Source: CAD feature listing. Evaluate the final solid. Frame: model axes, mm. A direction names the side the tool comes from. Give positions to 0.01 mm unless a question says otherwise; leave off trailing zeros. Order: outer loops, then holes, each group sorted by start corner. A loop starts at its lowest first (then second) coordinate and runs counter-clockwise, first axis right, second up. Notation, with made-up numbers: (-6.5, 23) -> (44.5, 23) arc R23 cw to (44.5, 37) -> close; hole circle Ø10 at (13.25, 59.25). An arc over 180 degrees is marked (long way). Answer in a Markdown table with one row per item.
```python
from build123d import *

# Parameters (mm, degrees)
F1_DEPTH  = 64
F2_R      = 60
F3_DEPTH  = 28.5
F4_R      = 60
F4_R_2    = 57
F5_DEPTH  = 25.5
F7_DEPTH  = 6.25
F8_R      = 13.15
F9_DEPTH  = 64.001
F10_R     = 11
F11_DEPTH = 12
F12_R     = 13.15
F13_DEPTH = 25
F14_R     = 7
F15_DEPTH = 57.751


with BuildPart() as f1:
    # F0 (on Front) → F1 (new body)
    with BuildSketch(Plane.XZ):
        with BuildLine():
            ThreePointArc((-32.5, -28), (-25.1776695297, -45.6776695297), (-7.5, -53))
            Line((-7.5, -53), (7.5, -53))
            ThreePointArc((7.5, -53), (25.1776695297, -45.6776695297), (32.5, -28))
            Line((32.5, -28), (32.5, 28))
            ThreePointArc((32.5, 28), (25.1776695297, 45.6776695297), (7.5, 53))
            Line((7.5, 53), (-7.5, 53))
            ThreePointArc((-7.5, 53), (-25.1776695297, 45.6776695297), (-32.5, 28))
            Line((-32.5, 28), (-32.5, -28))
        make_face()
    extrude(amount=F1_DEPTH)

    # F2 (on face) → F3 (join)
    with BuildSketch(Plane.XZ.offset(64)):
        Circle(F2_R)
    extrude(amount=-F3_DEPTH)

    # F4 (on face) → F5 (cut)
    with BuildSketch(Plane.XZ.offset(64)):
        Circle(F4_R)
        Circle(F4_R_2, mode=Mode.SUBTRACT)
    extrude(amount=-F5_DEPTH, mode=Mode.SUBTRACT)

    # F6 (on face) → F7 (cut)
    with BuildSketch(Plane(origin=(0, 0, 0), x_dir=(-1, 0, 0), z_dir=(0, 1, 0))):
        with BuildLine():
            ThreePointArc((10.955166333, 46.2427935703), (16.0339049992, 39.9945133997), (17.85, 32.15))
            ThreePointArc((17.85, 32.15), (-7.8445133997, 16.1160950008), (-10.955166333, 46.2427935703))
            ThreePointArc((-10.955166333, 46.2427935703), (-10.6670838439, 46.4620865798), (-10.3746129282, 46.6754916127))
            add(Edge.make_bspline(
                [(-11.4193501695, 49.6480644458), (-9.7061666222, 49.8827470388), (-8.574372674, 48.2387921733), (-10.3746129282, 46.6754916127)],
                knots=[0, 0, 0, 0, 3.1442100344, 3.1442100344, 3.1442100344, 3.1442100344], degree=3))
            ThreePointArc((-11.4193501695, 49.6480644458), (-24.3852850691, 42.1027354841), (-29.5, 28))
            Line((-29.5, 28), (-29.5, -28))
            ThreePointArc((-29.5, -28), (-24.3852850691, -42.1027354841), (-11.4193501695, -49.6480644458))
            add(Edge.make_bspline(
                [(-11.4193501695, -49.6480644458), (-9.7061666222, -49.8827470388), (-8.574372674, -48.2387921733), (-10.3746129282, -46.6754916127)],
                knots=[0, 0, 0, 0, 3.1442100344, 3.1442100344, 3.1442100344, 3.1442100344], degree=3))
            ThreePointArc((-10.3746129282, -46.6754916127), (-10.6670838439, -46.4620865798), (-10.955166333, -46.2427935703))
            ThreePointArc((-10.955166333, -46.2427935703), (-7.8445133997, -16.1160950008), (17.85, -32.15))
            ThreePointArc((17.85, -32.15), (16.0339049992, -39.9945133997), (10.955166333, -46.2427935703))
            ThreePointArc((10.955166333, -46.2427935703), (10.6670838439, -46.4620865798), (10.3746129282, -46.6754916127))
            add(Edge.make_bspline(
                [(11.4193501695, -49.6480644458), (9.7061666222, -49.8827470388), (8.574372674, -48.2387921733), (10.3746129282, -46.6754916127)],
                knots=[0, 0, 0, 0, 3.1442100344, 3.1442100344, 3.1442100344, 3.1442100344], degree=3))
            ThreePointArc((11.4193501695, -49.6480644458), (24.3852850691, -42.1027354841), (29.5, -28))
            Line((29.5, -28), (29.5, 28))
            ThreePointArc((29.5, 28), (24.3852850691, 42.1027354841), (11.4193501695, 49.6480644458))
            add(Edge.make_bspline(
                [(11.4193501695, 49.6480644458), (9.7061666222, 49.8827470388), (8.574372674, 48.2387921733), (10.3746129282, 46.6754916127)],
                knots=[0, 0, 0, 0, 3.1442100344, 3.1442100344, 3.1442100344, 3.1442100344], degree=3))
            ThreePointArc((10.3746129282, 46.6754916127), (10.6670838439, 46.4620865798), (10.955166333, 46.2427935703))
        make_face()
    extrude(amount=-F7_DEPTH, mode=Mode.SUBTRACT)

    # F8 (on face) → F9 (cut, through all)
    with BuildSketch(Plane(origin=(0, 0, 0), x_dir=(-1, 0, 0), z_dir=(0, 1, 0))):
        with Locations((0, 32.15)):
            Circle(F8_R)
        with Locations((0, -32.15)):
            Circle(F8_R)
    extrude(amount=-F9_DEPTH, mode=Mode.SUBTRACT)

    # F10 (on face) → F11 (cut)
    with BuildSketch(Plane(origin=(0, -6.25, 0), x_dir=(-1, 0, 0), z_dir=(0, 1, 0))):
        with BuildLine():
            add(Edge.make_bspline(
                [(11.4193501695, -49.6480644458), (9.7061666222, -49.8827470388), (8.574372674, -48.2387921733), (10.3746129282, -46.6754916127)],
                knots=[0, 0, 0, 0, 3.1442100344, 3.1442100344, 3.1442100344, 3.1442100344], degree=3))
            ThreePointArc((11.4193501695, -49.6480644458), (24.3852850691, -42.1027354841), (29.5, -28))
            Line((29.5, -28), (29.5, 28))
            ThreePointArc((29.5, 28), (24.3852850691, 42.1027354841), (11.4193501695, 49.6480644458))
            add(Edge.make_bspline(
                [(11.4193501695, 49.6480644458), (9.7061666222, 49.8827470388), (8.574372674, 48.2387921733), (10.3746129282, 46.6754916127)],
                knots=[0, 0, 0, 0, 3.1442100344, 3.1442100344, 3.1442100344, 3.1442100344], degree=3))
            ThreePointArc((10.3746129282, 46.6754916127), (0.3620324059, 14.3036717351), (-10.955166333, 46.2427935703))
            ThreePointArc((-10.955166333, 46.2427935703), (-10.6670838439, 46.4620865798), (-10.3746129282, 46.6754916127))
            add(Edge.make_bspline(
                [(-11.4193501695, 49.6480644458), (-9.7061666222, 49.8827470388), (-8.574372674, 48.2387921733), (-10.3746129282, 46.6754916127)],
                knots=[0, 0, 0, 0, 3.1442100344, 3.1442100344, 3.1442100344, 3.1442100344], degree=3))
            ThreePointArc((-11.4193501695, 49.6480644458), (-24.3852850691, 42.1027354841), (-29.5, 28))
            Line((-29.5, 28), (-29.5, -28))
            ThreePointArc((-29.5, -28), (-24.3852850691, -42.1027354841), (-11.4193501695, -49.6480644458))
            add(Edge.make_bspline(
                [(-11.4193501695, -49.6480644458), (-9.7061666222, -49.8827470388), (-8.574372674, -48.2387921733), (-10.3746129282, -46.6754916127)],
                knots=[0, 0, 0, 0, 3.1442100344, 3.1442100344, 3.1442100344, 3.1442100344], degree=3))
            ThreePointArc((-10.3746129282, -46.6754916127), (0, -14.3), (10.3746129282, -46.6754916127))
        make_face()
        Circle(F10_R, mode=Mode.SUBTRACT)
    extrude(amount=-F11_DEPTH, mode=Mode.SUBTRACT)

    # F12 (on face) → F13 (cut)
    with BuildSketch(Plane.XZ.offset(64)):
        with BuildLine():
            ThreePointArc((-53.1616791792, 2.8478205157), (-50.6283325618, 2.8655619516), (-48.9143201794, 1))
            Line((-48.9143201794, 1), (-26.9143201794, 1))
            Line((-26.9143201794, 1), (-26.9143201794, -1))
            Line((-26.9143201794, -1), (-48.9143201794, -1))
            ThreePointArc((-48.9143201794, -1), (-50.6283325618, -2.8655619516), (-53.1616791792, -2.8478205157))
            Line((-53.1616791792, -2.8478205157), (-54.7518743997, -5.2184528093))
            ThreePointArc((-54.7518743997, -5.2184528093), (0, -55), (54.7518743997, -5.2184528093))
            Line((54.7518743997, -5.2184528093), (53.1616791792, -2.8478205157))
            ThreePointArc((53.1616791792, -2.8478205157), (50.6283325618, -2.8655619516), (48.9143201794, -1))
            Line((48.9143201794, -1), (26.9143201794, -1))
            Line((26.9143201794, -1), (26.9143201794, 1))
            Line((26.9143201794, 1), (48.9143201794, 1))
            ThreePointArc((48.9143201794, 1), (50.6283325618, 2.8655619516), (53.1616791792, 2.8478205157))
            Line((53.1616791792, 2.8478205157), (54.7518743997, 5.2184528093))
            ThreePointArc((54.7518743997, 5.2184528093), (0, 55), (-54.7518743997, 5.2184528093))
            Line((-54.7518743997, 5.2184528093), (-53.1616791792, 2.8478205157))
        make_face()
        with Locations((0, -32.15)):
            Circle(F12_R, mode=Mode.SUBTRACT)
        with Locations((0, 32.15)):
            Circle(F12_R, mode=Mode.SUBTRACT)
    extrude(amount=-F13_DEPTH, mode=Mode.SUBTRACT)

    # F14 (on face) → F15 (cut, through all)
    with BuildSketch(Plane(origin=(0, -6.25, 0), x_dir=(-1, 0, 0), z_dir=(0, 1, 0))):
        Circle(F14_R)
    extrude(amount=-F15_DEPTH, mode=Mode.SUBTRACT)


solid = f1.part
```
(1) Access query for faces 1 (the cylindrical face through (-24.247, -8.997, -42.267)), 2 (the flat face through (-38, -52, 1)), 3 (the cylindrical face through (-25.371, -17.502, -45.482)), 4 (the flat face through (-32.5, -18, 0)). Directions: +Z, -Z, +X, -X, +Y, -Y. A direction counts if a zero-diameter tool reaches every point of the face in a straight line with its end or side. Return the directions, or none.
A:
| item | result |
|---|---|
| face 1 | +Y |
| face 2 | -Y |
| face 3 | -Z, -X, +Y |
| face 4 | +Z, -Z, -X, +Y |
(2) Section query C-C (z = -16). Return the cut outline in (x, y), plus the area to 3 significant figures.
A:
| item | result |
|---|---|
| outline | (-57.83, -38.5) -> (-54.71, -38.5) -> (-54.71, -64) -> (-52.62, -64) -> (-52.62, -39) -> (52.62, -39) -> (52.62, -64) -> (54.71, -64) -> (54.71, -38.5) -> (57.83, -38.5) -> (57.83, -35.5) -> (32.5, -35.5) -> (32.5, 0) -> (29.5, 0) -> (29.5, -18.25) -> (7.6, -18.25) -> (7.6, 0) -> (-7.6, 0) -> (-7.6, -18.25) -> (-29.5, -18.25) -> (-29.5, 0) -> (-32.5, 0) -> (-32.5, -35.5) -> (-57.83, -35.5) -> close |
| area | 2,010 mm^2 |
(3) Pull-direction query (Z, two-part tool) for faces 5 (the flat face through (22, -38.5, -53)), 6 (the cylindrical face through (-24.52, -9, 41.94)), 7 (the flat face through (0, -18, -53)); classes: +Z half, -Z half, draft (parallel to the pull), parting line (faces both ways), or undercut.
A:
| item | result |
|---|---|
| face 5 | draft |
| face 6 | undercut |
| face 7 | -Z half |
(4) First-contact query: pin 1 Ø11 at (x, z) = (2.5, -4) entering from +Y; pin 2 Ø3 at (x, z) = (32, 30) entering from -Y; pin 3 Ø8 at (y, z) = (-27, -46.5) entering from +X; pin 4 Ø21 at (x, z) = (0, -32.15) entering from -Y. Flat tips, straight axial feed; report the tip coordinate or a pass-through.
A:
| item | result |
|---|---|
| pin 1 | stops at y = -6.25 |
| pin 2 | stops at y = -39 |
| pin 3 | stops at x = 27.87 |
| pin 4 | passes through |
(5) Section query B-B (x = 0). Give the number of separate pieces and of enclosed holes in the cut face, plus the area to 3 significant figures.
A:
| item | result |
|---|---|
| separate pieces | 4 |
| enclosed holes | 0 |
| area | 1,510 mm^2 |
(6) Section query A-A (z = 32.15). Return the cut outline in (x, y), plus the area to 3 significant figures.
A:
| item | result |
|---|---|
| outline | (-50.66, -38.5) -> (-47.07, -38.5) -> (-47.07, -64) -> (-44.62, -64) -> (-44.62, -39) -> (-13.15, -39) -> (-13.15, 0) -> (-17.85, 0) -> (-17.85, -18.25) -> (-29.11, -18.25) -> (-29.11, 0) -> (-32.15, 0) -> (-32.15, -35.5) -> (-50.66, -35.5) -> close; (13.15, -39) -> (44.62, -39) -> (44.62, -64) -> (47.07, -64) -> (47.07, -38.5) -> (50.66, -38.5) -> (50.66, -35.5) -> (32.15, -35.5) -> (32.15, 0) -> (29.11, 0) -> (29.11, -18.25) -> (17.85, -18.25) -> (17.85, 0) -> (13.15, 0) -> close |
| area | 1,320 mm^2 |
(7) Ray query, probe 1 along Z at (x, y) = (0, -20); probe 2 along Z at (x, y) = (0, -14); probe 3 along Z at (x, y) = (-5.5, -36). Return the intervals inside material, ascending.
A:
| item | result |
|---|---|
| probe 1 | z = -53 to -45.3, -19 to -7, 7 to 19, 45.3 to 53 |
| probe 2 | z = -53 to -45.3, -19 to -14.3, -11 to -7, 7 to 11, 14.3 to 19, 45.3 to 53 |
| probe 3 | z = -59.75 to -44.09, -20.21 to -4.33, 4.33 to 20.21, 44.09 to 59.75 |
